```python
from build123d import *

# Parameters (mm, degrees)
F0_R      = 11.1125
F0_R_2    = 4.7625
F1_DEPTH  = 46.99
F2_W      = 46.99
F2_H      = 7.62
F3_DEPTH  = 38.1
F3_FACE_W = 46.99
F3_FACE_H = 7.62
F4_DEPTH  = 3.556
F5_R      = 0.79375
F6_DEPTH  = 25.4
F7_R      = 4.92125
F8_DEPTH  = 25.4
F10_DEPTH = 46.991


with BuildPart() as f1:
    # F0 (on Front) → F1 (new body)
    with BuildSketch(Plane.XZ):
        Circle(F0_R)
        Circle(F0_R_2, mode=Mode.SUBTRACT)
    extrude(amount=F1_DEPTH)

    # F2 (on Right) → F3 (join)
    with BuildSketch(Plane.YZ):
        with Locations((-23.495, 0)):
            Rectangle(F2_W, F2_H)
    extrude(amount=-F3_DEPTH)

    # F3_face (on face) → F4 (cut)
    with BuildSketch(Plane(origin=(0, -23.495, 0), x_dir=(0, 1, 0), z_dir=(1, 0, 0))):
        Rectangle(F3_FACE_W, F3_FACE_H)
    extrude(amount=-F4_DEPTH, mode=Mode.SUBTRACT)

    # F5 (on Top) → F6 (cut)
    with BuildSketch(Plane.XY):
        with Locations((0, -7.62)):
            Circle(F5_R)
        with Locations((0, -39.37)):
            Circle(F5_R)
    extrude(amount=-F6_DEPTH, mode=Mode.SUBTRACT)

    # F7 (on Right) → F8 (cut)
    with BuildSketch(Plane.YZ):
        with Locations((-23.495, 0)):
            Circle(F7_R)
    extrude(amount=F8_DEPTH, mode=Mode.SUBTRACT)

    # F9 (on face) → F10 (cut, through all)
    with BuildSketch(Plane(origin=(0, 0, 0), x_dir=(-1, 0, 0), z_dir=(0, 1, 0))):
        with BuildLine():
            ThreePointArc((2.8575, 3.81), (-4.7625, 0), (2.8575, -3.81))
            ThreePointArc((2.8575, -3.81), (4.259709, -2.129855), (4.7625, 0))
            ThreePointArc((4.7625, 0), (4.259709, 2.129855), (2.8575, 3.81))
        make_face()
    extrude(amount=-F10_DEPTH, mode=Mode.SUBTRACT)


solid = f1.part
```
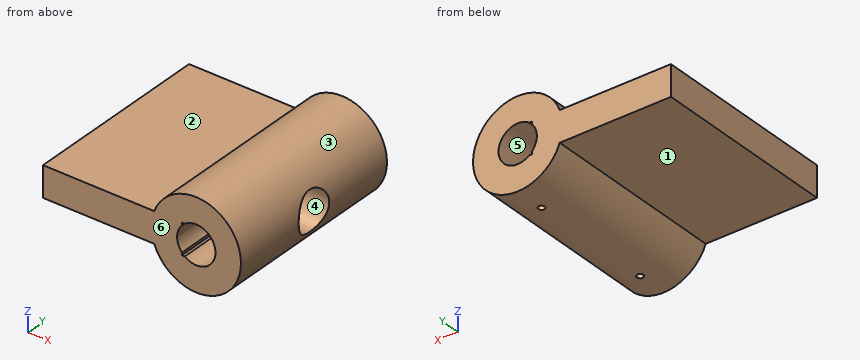
Could you check a few things on this model? Use its own coordinates, in mm. Face numbers are marked on the shaded views. A direction names the side the tool comes from. Coordinates: 2 decimals unless noted, no trailing zeros. Write each loop counter-clockwise with the first axis right and the second up, starting at its lowest first coordinate (ties: lowest second). Pieces come first, ordered by that corner, then holes. Notation, with made-up numbers: (27.5, 89.25) -> (43.5, 89.25) arc R22 ccw to (43.5, 128.25) -> close; hole circle Ø5 at (78, -4.75). An arc over 180 degrees is marked (long way). One line per question, with ' | ' between items. Start each with the question number.
1. If we section it at C-C (z = -6.75): Please give me the cut outline in (x, y).
2. If we section it at B-B (z = 1): Please give me the cut outline in (x, y).
3. For the marked faces 1, 2 and 3, which set-ups out of +Z, -Z, +X, -X, +Y, -Y let a thin tool reach every point of the face, with its end or its side?
4. Thinking about a two-plate mould opening in Y: for the marked faces 4, 5 and 6, which applies, pulls with the +Y half, pulls with the -Y half, needs draft (parallel to the pull), parting line crosses it, or undercut?
5. If we section it at A-A (y = -35.5): Please give me the cut outline in (x, z) (1 decimal), and give its area (3 significant figures).
6. Will these pins go through, and if not, where does the flat tip stop? P1, Ø5, axis at x = -12.5, y = -33, coming from the +Z side; P2, Ø1, axis at x = -32.5, y = -6, coming from the +Z side; P3, Ø0.8, axis at x = -3.5, y = -19, coming from the +Z side; P4, Ø6, axis at x = -14, z = -7.5, coming from the -Y side.
7. Please list where these lines run through material, in increasing order: line 1 along X through (y, z) = (-33.5, 0); line 2 along Y through (x, z) = (7, 0); line 3 along Z through (x, y) = (0, -25).
8. If we section it at D-D (x = -13): Please give me the cut outline in (y, z).
Return value:
1) outline: (-8.83, -46.99) -> (8.83, -46.99) -> (8.83, 0) -> (-8.83, 0) -> close; hole circle Ø1.59 at (0, -39.37); hole circle Ø1.59 at (0, -7.62)
2) outline: (-38.1, -46.99) -> (-4.66, -46.99) -> (-4.66, 0) -> (-38.1, 0) -> close; (4.66, -46.99) -> (11.07, -46.99) -> (11.07, -28.31) -> (4.66, -28.31) -> close; (4.66, -18.68) -> (11.07, -18.68) -> (11.07, 0) -> (4.66, 0) -> close
3) face 1: -Z, -X, +Y, -Y | face 2: +Z, -X, +Y, -Y | face 3: +Y, -Y
4) face 4: undercut | face 5: needs draft | face 6: pulls with the -Y half
5) outline: (-38.1, -3.8) -> (-10.4, -3.8) arc R11.1 ccw (long way) to (-10.4, 3.8) -> (-38.1, 3.8) -> close; hole (-4.8, 0) arc R4.8 ccw to (-3.6, -3.2) -> (-3.6, -3.8) -> (-2.9, -3.8) arc R4.8 ccw (long way) to (-2.9, 3.8) -> (-3.6, 3.8) -> (-3.6, 3.2) arc R4.8 ccw to start | area: 524 mm²
6) P1: stops at z = 4.85 | P2: stops at z = 3.81 | P3: stops at z = 10.67 | P4: passes through
7) line 1: x = -38.1 to -4.76, 4.76 to 11.11 | line 2: y = -46.99 to -28.42, -18.57 to 0 | line 3: z = -11.11 to -4.76, 4.76 to 11.11
8) outline: (-46.99, -3.81) -> (0, -3.81) -> (0, 3.81) -> (-46.99, 3.81) -> close
